Autodesk Inventor part; units mm, degrees
ref_plane "YZ Plane" through (0, 0, 0) normal (1, 0, 0) x (0, 1, 0)
ref_plane "XZ Plane" through (0, 0, 0) normal (0, 1, 0) x (-1, 0, 0)
ref_plane "XY Plane" through (0, 0, 0) normal (0, 0, 1) x (1, 0, 0)
sketch "Sketch1" plane through (0, 0, 0) normal (0, 1, 0) x (-1, 0, 0)
  circle A0 centre (0, 0) radius 25.4 construction
  line L0 (-25.4, -25.4) -> (25.4, -25.4)
  line L1 (25.4, -25.4) -> (25.4, 25.4)
  line L2 (25.4, 25.4) -> (-25.4, 25.4)
  line L3 (-25.4, 25.4) -> (-25.4, -25.4)
  line L4 (-25.4, -25.4) -> (25.4, 25.4) construction
  line L5 (25.4, -25.4) -> (-25.4, 25.4) construction
  dimension "d0" = 50.8
  dimension "d1" = 50.8
extrude "Extrusion1" add sketch "Sketch1" along normal blind 76.2
sketch "Sketch3" plane through (0, 0, 0) normal (1, 0, 0) x (0, 1, 0)
  line L0 (-43.9941, 0) -> (0, 25.4) construction
  line L1 (0, -25.4) -> (0, 25.4) construction
  line L2 (76.2, 25.4) -> (0, 25.4) construction
  line L3 (0, 25.4) -> (0, 0) construction
  line L4 (-43.9941, 0) -> (0, 0) construction
  line L5 (-43.9941, 0) -> (0, -25.4) construction
  line L6 (98.9867, 82.55) -> (105.3367, 71.5515)
  line L7 (105.3367, 71.5515) -> (76.2, 54.7294)
  line L8 (76.2, 54.7294) -> (76.2, 25.4)
  line L9 (0, 25.4) -> (98.9867, 82.55)
  line L10 (0, 25.4) -> (76.2, 25.4)
  dimension "d14" = 60
  dimension "d15" = 12.7
  dimension "d16" = 114.3
extrude "Extrusion2" add sketch "Sketch3" along normal mid plane 50.8
pattern_circular "Circular Pattern1" count 4 over 360 about axis through (0, -10, 0) along (0, 1, 0) of "Extrusion2"
properties part number "4-Tool_Head"
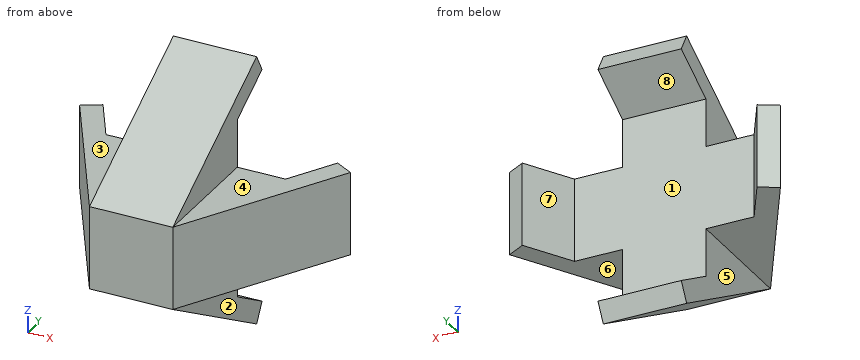
The listing builds one solid part. Answer for the finished solid, in the listing's coordinates (mm). Face numbers are marked on the shaded views. A direction names the side the tool comes from. Give positions to 0.01 mm unless a question says otherwise; leave off trailing zeros. Order: outer loops, then holes, each group sorted by start corner. A loop starts at its lowest first (then second) coordinate and runs counter-clockwise, first axis right, second up. Notation, with made-up numbers: (-15, 44.25) - (28, 44.25) arc R14 ccw to (28, 48.25) - close; hole circle Ø3 at (-8, 9). An arc over 180 degrees is marked (long way). One line per item, written item: value. Start each with the question number.
1) A cutting plane is placed at B-B on x = -5.5. Give the vertices of the cut face in (y, z).
2) A tool of negligible diameter and unlimited length cuts with its end or side. For the marked faces 1, 2, 3, 4 and 5, from which of +Z, -Z, +X, -X, +Y, -Y can it reach the whole face along a straight path? Write none if from no direction.
3) A cutting plane is placed at C-C on z = -14. Give the vertices of the cut face in (x, y), then the cut area to 3 significant figures.
4) Given pin 1 Ø10 at (x, y) = (-28.5, 62.5) entering from +Z; pin 2 Ø3 at (y, z) = (24.5, -10.5) entering from +X; pin 3 Ø4 at (x, z) = (-35.5, 23.5) entering from +Y, each flat-ended and moving along its own axis, determine where each tip first touches the part or whether it passes through.
5) A cutting plane is placed at D-D on y = 47.5. Give the vertices of the cut face in (x, z), then the cut area to 3 significant figures.
6) Find the intervals of material crossed by L1, parallel to X at y = 63.5, z = 28; L2, parallel to Y at x = -17, z = 7; L3, parallel to Y at x = -39.5, z = 22.5, in increasing order.
7) The mould has two halves that part along Z. Classify the marked faces 6, 7 and 8: released by +Z, released by -Z, zero draft, split by the parting line, or undercut.
8) A cutting plane is placed at A-A on y = 92.5. Give the vertices of the cut face in (x, z).
Answer sheet:
1. outline: (0, -25.4) - (98.99, -82.55) - (105.34, -71.55) - (76.2, -54.73) - (76.2, 54.73) - (105.34, 71.55) - (98.99, 82.55) - (0, 25.4) - close
2. face 1: +Y
2. face 2: -Z, +X, +Y, -Y
2. face 3: +Z, -X, +Y, -Y
2. face 4: +Z, +X, +Y, -Y
2. face 5: -Z, -X, +Y, -Y
3. outline: (-82.55, 98.99) - (-25.4, 0) - (25.4, 0) - (82.55, 98.99) - (71.55, 105.34) - (54.73, 76.2) - (-54.73, 76.2) - (-71.55, 105.34) - close
3. area: 7,980 mm2
4. pin 1: stops at z = 63.75
4. pin 2: stops at x = 40.41
4. pin 3: stops at y = 76.2
5. outline: (-52.82, -25.4) - (-25.4, -25.4) - (-25.4, -52.82) - (25.4, -52.82) - (25.4, -25.4) - (52.82, -25.4) - (52.82, 25.4) - (25.4, 25.4) - (25.4, 52.82) - (-25.4, 52.82) - (-25.4, 25.4) - (-52.82, 25.4) - close
5. area: 8,150 mm2
6. L1: x = -25.4 to 25.4
6. L2: y = 0 to 76.2
6. L3: y = 24.42 to 76.2
7. face 6: released by -Z
7. face 7: zero draft
7. face 8: undercut
8. outline: (-78.8, -25.4) - (-64.14, -25.4) - (-64.14, 25.4) - (-78.8, 25.4) - close; (-25.4, -78.8) - (25.4, -78.8) - (25.4, -64.14) - (-25.4, -64.14) - close; (-25.4, 64.14) - (25.4, 64.14) - (25.4, 78.8) - (-25.4, 78.8) - close; (64.14, -25.4) - (78.8, -25.4) - (78.8, 25.4) - (64.14, 25.4) - close
